```python
from build123d import *

# Parameters (mm, degrees)
BOSS_EXTRUDE1_DEPTH = 5
BOSS_EXTRUDE2_DEPTH = 185
BOSS_EXTRUDE3_DEPTH = 5
FILLET1_R           = 10
FILLET2_R           = 2


with BuildPart() as part:
    # Sketch1 → Boss-Extrude1 (new body)
    with BuildSketch(Plane.XY):
        with BuildLine():
            Line((-145, 20), (-145, -20))
            Line((-145, -20), (145, -20))
            Line((145, -20), (145, 20))
            Line((145, 20), (15, 20))
            ThreePointArc((15, 20), (0, 5), (-15, 20))
            Line((-15, 20), (-145, 20))
        make_face()
    extrude(amount=-BOSS_EXTRUDE1_DEPTH)

    # Sketch2 → Boss-Extrude2 (add)
    with BuildSketch(Plane(origin=(0, 0, -5), x_dir=(-1, 0, 0), z_dir=(0, 0, -1))):
        Polygon((-140, -15), (-140, 15), (-140, 20), (-145, 20), (-145, -20), (145, -20), (145, 20), (140, 20), (140, 15), (140, -15), align=None)
    extrude(amount=BOSS_EXTRUDE2_DEPTH)

    # Sketch3 → Boss-Extrude3 (add)
    with BuildSketch(Plane(origin=(0, 0, -190), x_dir=(-1, 0, 0), z_dir=(0, 0, -1))):
        with BuildLine():
            Line((140, -15), (140, 20))
            Line((140, 20), (15, 20))
            ThreePointArc((15, 20), (0, 5), (-15, 20))
            Line((-15, 20), (-140, 20))
            Line((-140, 20), (-140, -15))
            Line((-140, -15), (140, -15))
        make_face()
        with BuildLine():
            ThreePointArc((-15, 20), (0, 5), (15, 20))
            Line((15, 20), (-15, 20))
        make_face()
        Polygon((145, 20), (140, 20), (140, -15), (-140, -15), (-140, 20), (-145, 20), (-145, -20), (145, -20), align=None)
    extrude(amount=BOSS_EXTRUDE3_DEPTH)

    # Fillet1
    fillet1_edges = [part.edges().sort_by_distance(p)[0] for p in [
        (145, -20, -97.5),
        (-145, -20, -97.5),
        (-15, 20, -2.5),
        (15, 20, -2.5),
        (-140, 2.5, -190),
        (140, 2.5, -190),
        (-140, 2.5, -5),
        (140, 2.5, -5),
        (145, 0, -195),
        (0, -20, -195),
        (-145, 0, -195),
        (145, 0, 0),
        (0, -20, 0),
        (-145, 0, 0),
    ]]
    fillet(fillet1_edges, radius=FILLET1_R)

    # Fillet2
    fillet2_edges = [part.edges().sort_by_distance(p)[0] for p in [
        (142.071067812, 20, -192.071067812),
        (-142.071067812, 20, -192.071067812),
        (142.071067812, 20, -2.928932188),
        (-142.071067812, 20, -2.928932188),
        (0, 20, -195),
        (-145, 20, -97.5),
        (145, 20, -97.5),
        (78.956439237, 20, 0),
        (0, 5, 0),
        (-78.956439237, 20, 0),
        (-17.4356529, 18.366600265, 0),
        (17.4356529, 18.366600265, 0),
    ]]
    fillet(fillet2_edges, radius=FILLET2_R)


solid = part.part
```
Can you work these out from the model? Positions are in its coordinate system, mm. A direction names the side the tool comes from. Round coordinates to 2 decimals unless told otherwise and drop trailing zeros. Loops run counter-clockwise (first coordinate to the right, second up) from the corner with the lowest first, then second, coordinate; pieces in that order, holes last. Notation, with made-up numbers: (42.5, 78.5) -> (80.5, 78.5) arc R34 cw to (80.5, 116.5) -> close; hole circle Ø2 at (-34, -21.5). An arc over 180 degrees is marked (long way). One line per item, written item: value. Start each with the question number.
1. If we section it at A-A, the plane y = 0: Write out the boundary of the cut face in (x, z), then the cut area to 3 significant figures.
2. If we section it at B-B, the plane x = 51.5: Write out the boundary of the cut face in (y, z).
3. If we section it at C-C, the plane z = -137.5: Write out the boundary of the cut face in (x, y), then the cut area to 3 significant figures.
4. For faces 1 (the flat face through (2, 4, -195)), 2 (the cylindrical face through (-137.15, 2.25, -186.99)), 3 (the cylindrical face through (-17.368, 18.322, -3.521)), which set-ups out of +Z, -Z, +X, -X, +Y, -Y let a thin tool reach every point of the face, with its end or its side?
5. For pin 1 (4 mm diameter, centred on x = -28, z = -132, fed in from +Y); pin 2 (6 mm diameter, centred on x = 48, y = -14.5, fed in from -Z), each with a flat end and sliding along its axis, tell me the tip position at first contact or that it passes through.
6. If I drill on probe 1 along Z at (x, y) = (-114, 14); probe 2 along X at (y, z) = (13.5, -43); probe 3 along Y at (x, z) = (-80, -143), over which ranges is the centre line in solid material (lowest first)?
7. If we mould it in two halves opening along X, with no side actions, what happens to faces 4 (the cylindrical face through (-1.89, -17.15, -191.99)), 5 (the cylindrical face through (-142.15, 4.2, -191.99)), 6 (the cylindrical face through (0, 5, -3))? For each: pulls with the +X half, pulls with the -X half, needs draft (parallel to the pull), parting line crosses it, or undercut.
Calculated:
1. outline: (-145, -185) arc R10 ccw to (-135, -195) -> (135, -195) arc R10 ccw to (145, -185) -> (145, -10) arc R10 ccw to (135, 0) -> (-135, 0) arc R10 ccw to (-145, -10) -> close; hole (-140, -180) arc R10 ccw to (-130, -190) -> (130, -190) arc R10 ccw to (140, -180) -> (140, -15) arc R10 ccw to (130, -5) -> (-130, -5) arc R10 ccw to (-140, -15) -> close
1. area: 4,750 mm²
2. outline: (-20, -185) arc R10 ccw to (-10, -195) -> (18, -195) arc R2 ccw to (20, -193) -> (20, -190) -> (-15, -190) -> (-15, -5) -> (20, -5) -> (20, -2) arc R2 ccw to (18, 0) -> (-10, 0) arc R10 ccw to (-20, -10) -> close
3. outline: (-145, -10) arc R10 ccw to (-135, -20) -> (135, -20) arc R10 ccw to (145, -10) -> (145, 18) arc R2 ccw to (143, 20) -> (140, 20) -> (140, -15) -> (-140, -15) -> (-140, 20) -> (-143, 20) arc R2 ccw to (-145, 18) -> close
3. area: 1,760 mm²
4. face 1: -Z, +X, -X, +Y, -Y
4. face 2: +Y
4. face 3: +Z, +Y
5. pin 1: stops at y = -15
5. pin 2: stops at z = -194.89
6. probe 1: z = -195 to -190, -5 to 0
6. probe 2: x = -145 to -140, 140 to 145
6. probe 3: y = -20 to -15
7. face 4: needs draft
7. face 5: pulls with the -X half
7. face 6: undercut
